The model under review builds one solid part; all positions refer to its coordinate system, in mm. A direction names the side the tool comes from. Round coordinates to 2 decimals unless told otherwise and drop trailing zeros. Order: outer loops, then holes, each group sorted by start corner. A loop starts at its lowest first (then second) coordinate and runs counter-clockwise, first axis right, second up.
1) Machinability: for faces 5 (the face through (1, -9.565, 15)), 6 (the face through (1, -2.785, 3)), 7 (the face through (-31, 7, 9.2)), which of the approach directions +Z, -Z, +X, -X, +Y, -Y give a long, thin tool a straight path to every point of the face, cutting with its end or side? Answer none if there is none.
2) Mouldability with a two-part tool opening along Z and no side actions: class faces 1 (the face through (-29.861, 7, 9)), 2 (the face through (-0.03, -10.07, -0.49)), 3 (the face through (1, 23.495, 10)), 4 (the face through (22.512, 15.613, 9.986)) as pulls with the +Z half, pulls with the -Z half, needs draft (parallel to the pull), parting line crosses it, or undercut.
3) To check wall thickness, follow L1, parallel to X at y = -1.5, z = 8.25; L2, parallel to Y at x = 1, z = 9.75; L3, parallel to Y at x = 16.5, z = 15.75. State the ranges of each line that lie inside material, in increasing order.
4) Consider section B-B (z = 8.2). Give the boundary of the cut face in (x, y).
5) Clearance check with flat-ended pins moving along their axes: P1, Ø1.2, axis at x = -31, y = 10, coming from the +Z side; P2, Ø1, axis at y = 3, z = 15, coming from the +X side; P3, Ø4.5, axis at x = -23, y = 16.5, coming from the +Z side. State where each tip first meets the part, or that it passes through.
6) Consider section D-D (z = 3.75). Give the boundary of the cut face in (x, y) (3 decimals).
Autodesk Inventor part; units mm, degrees
ref_plane "YZ Plane" through (0, 0, 0) normal (1, 0, 0) x (0, 1, 0)
ref_plane "XZ Plane" through (0, 0, 0) normal (0, 1, 0) x (-1, 0, 0)
ref_plane "XY Plane" through (0, 0, 0) normal (0, 0, 1) x (1, 0, 0)
sketch "Sketch1" plane through (0, 0, 0) normal (0, 0, 1) x (1, 0, 0)
  line L0 (-31.3608, 24.9952) -> (32.1392, 24.9952)
  line L1 (32.1392, 24.9952) -> (32.1392, -10.5648)
  line L2 (32.1392, -10.5648) -> (-31.3608, -10.5648)
  line L3 (-31.3608, -10.5648) -> (-31.3608, 24.9952)
  line L4 (30.6392, 23.4952) -> (-29.8608, 23.4952)
  line L5 (-29.8608, 23.4952) -> (-29.8608, -9.0648)
  line L6 (-29.8608, -9.0648) -> (30.6392, -9.0648)
  line L7 (30.6392, -9.0648) -> (30.6392, 23.4952)
  point P0 (0, 0)
  dimension "d0" = 63.5
  dimension "d1" = 35.56
  dimension "d2" = 1.5
extrude "Extrusion1" add sketch "Sketch1" along normal blind 16.2
sketch "Sketch2" plane through (0, 0, 0) normal (0, 0, -1) x (-1, 0, 0)
  line L0 (-32.1392, -10.5648) -> (31.3608, -10.5648)
  line L1 (31.3608, -10.5648) -> (31.3608, 24.9952)
  line L2 (31.3608, 24.9952) -> (-32.1392, 24.9952)
  line L3 (-32.1392, 24.9952) -> (-32.1392, -10.5648)
  point P0 (0, 0)
extrude "Extrusion2" add sketch "Sketch2" along normal blind 1.5
sketch "Sketch3" plane through (0, 0, 0) normal (0, 0, 1) x (1, 0, 0)
  line L0 (-18.6108, 17.2152) -> (19.3892, 17.2152)
  line L1 (19.3892, 17.2152) -> (19.3892, -2.7848)
  line L2 (19.3892, -2.7848) -> (-18.6108, -2.7848)
  line L3 (-18.6108, -2.7848) -> (-18.6108, 17.2152)
  line L4 (30.6392, -9.0648) -> (-29.8608, -9.0648)
  line L5 (-29.8608, 23.4952) -> (30.6392, 23.4952)
  line L6 (30.6392, 23.4952) -> (30.6392, -9.0648)
  line L7 (30.6392, -9.0648) -> (30.6392, 23.4952)
  line L8 (30.6392, 23.4952) -> (-29.8608, 23.4952)
  line L9 (-29.8608, 23.4952) -> (-29.8608, -9.0648)
  line L10 (-29.8608, -9.0648) -> (30.6392, -9.0648)
  point P0 (0, 0)
  dimension "d7" = 38
  dimension "d8" = 20
  dimension "d9" = 6.28
  dimension "d10" = 32.56
  dimension "d11" = 11.25
  dimension "d12" = 60.5
extrude "Extrusion3" add sketch "Sketch3" along normal blind 6
sketch "Sketch4" plane through (0, 0, 6) normal (0, 0, 1) x (1, 0, 0)
  circle A0 centre (-22.4708, 16.1052) radius 1
  circle A1 centre (-22.4708, -1.6748) radius 1
  circle A2 centre (23.2492, -1.6748) radius 1
  circle A3 centre (23.2489, 16.2887) radius 1
  line L0 (30.6392, -9.0648) -> (-29.8608, -9.0648)
  line L1 (-29.8608, 23.4952) -> (30.6392, 23.4952)
  line L2 (-29.8608, -9.0648) -> (-29.8608, 23.4952)
  point P0 (0, 0)
  dimension "d15" = 2
  dimension "d16" = 2
  dimension "d17" = 2
  dimension "d18" = 2
  dimension "d19" = 45.72
  dimension "d20" = 45.72
  dimension "d21" = 17.78
  dimension "d22" = 7.39
  dimension "d23" = 32.56
  dimension "d24" = 60.5
  dimension "d25" = 7.39
  dimension "d26" = 0
extrude "Extrusion4" add sketch "Sketch4" along normal blind 5
sketch "Sketch5" plane through (0, 0, 6) normal (0, 0, 1) x (1, 0, 0)
  circle A0 centre (-22.4708, 16.1052) radius 1
  circle A1 centre (-22.4708, -1.6748) radius 1
  circle A2 centre (23.2492, -1.6748) radius 1
  circle A3 centre (23.2489, 16.2887) radius 1
  circle A4 centre (-22.4708, 16.1052) radius 2
  circle A5 centre (-22.4708, -1.6748) radius 2
  circle A6 centre (23.2492, -1.6748) radius 2
  circle A7 centre (23.2489, 16.2887) radius 2
  point P0 (0, 0)
  dimension "d29" = 1
  dimension "d30" = 1
  dimension "d31" = 1
  dimension "d32" = 1
extrude "Extrusion5" add sketch "Sketch5" along normal blind 3
fillet "Fillet1" radius 1.5 4 edges at (-31.3608, -10.5648, 7.35) (32.1392, -10.5648, 7.35) (32.1392, 24.9952, 7.35) (-31.3608, 24.9952, 7.35)
sketch "Sketch6" plane through (32.1392, -9.0648, 16.2) normal (1, 0, 0) x (0, 0, -1)
  circle A0 centre (8, 16.28) radius 3.2
  line L0 (0, 0) -> (0, 32.56)
  line L1 (0, -1.5) -> (17.7, -1.5)
  line L2 (17.7, 34.06) -> (0, 34.06)
  point P0 (16.2, 9.0648)
  dimension "d36" = 6.4
  dimension "d37" = 8
  dimension "d38" = 17.78
  dimension "d39" = 35.56
extrude "Extrusion6" cut sketch "Sketch6" against normal up to surface (12.75 mm away)
sketch "Sketch7" plane through (19.3892, -2.7848, 0) normal (-1, 0, 0) x (0, 0, 1)
  arc A0 (6, 12.3238) -> (6, 7.6762) centre (8.2, 10) ccw
  circle A1 centre (8.2, 10) radius 5.5
  point P0 (0, 2.7848)
  dimension "d42" = 11
extrude "Extrusion7" cut sketch "Sketch7" against normal up to surface (11.25 mm away)
sketch "Sketch8" plane through (0, 0, 6) normal (0, 0, 1) x (1, 0, 0)
  line L0 (-18.6108, -2.7848) -> (-18.6108, 17.2152)
  line L1 (-18.6108, 2.4694) -> (-22.595, 2.4694)
  line L2 (-22.595, 2.4694) -> (-22.595, 12.7792)
  line L3 (-22.595, 12.7792) -> (-18.6108, 12.7792)
  line L4 (-18.6108, 12.7792) -> (-18.6108, 2.4694)
  point P0 (0, 0)
extrude "Extrusion8" cut sketch "Sketch8" against normal up to surface (6 mm away)
chamfer "Chamfer1" distance 2 angle 45 2 edges at (-18.6108, 2.4694, 3) (-18.6108, 12.7792, 3)
chamfer "Chamfer2" distance 4 angle 45 1 edges at (-22.595, 7.6243, 6)
sketch "Sketch9" plane through (0, 0, 16.2) normal (0, 0, 1) x (1, 0, 0)
  line L0 (-29.8608, 23.4952) -> (30.6392, 23.4952)
  line L1 (-29.8608, -9.0648) -> (-29.8608, 23.4952)
  line L2 (30.6392, -9.0648) -> (-29.8608, -9.0648)
  line L3 (30.6392, 23.4952) -> (30.6392, -9.0648)
  line L4 (29.6392, 22.4952) -> (-28.8608, 22.4952)
  line L5 (-28.8608, 22.4952) -> (-28.8608, -8.0648)
  line L6 (-28.8608, -8.0648) -> (29.6392, -8.0648)
  line L7 (29.6392, -8.0648) -> (29.6392, 22.4952)
  point P0 (0, 0)
  dimension "d53" = 1
extrude "Extrusion9" add sketch "Sketch9" against normal blind 3
chamfer "Chamfer3" distance 1 angle 45 4 edges at (-28.8608, 7.2152, 13.2) (0.3892, 22.4952, 13.2) (0.3892, -8.0648, 13.2) (29.6392, 7.2152, 13.2)
sketch "Sketch10" plane through (0, 0, 16.2) normal (0, 0, 1) x (1, 0, 0)
  line L0 (30.6392, 24.9952) -> (-29.8608, 24.9952)
  arc A0 (-29.8608, 24.9952) -> (-31.3608, 23.4952) centre (-29.8608, 23.4952) ccw
  line L1 (-31.3608, 23.4952) -> (-31.3608, -9.0648)
  arc A1 (-31.3608, -9.0648) -> (-29.8608, -10.5648) centre (-29.8608, -9.0648) ccw
  line L2 (-29.8608, -10.5648) -> (30.6392, -10.5648)
  arc A2 (30.6392, -10.5648) -> (32.1392, -9.0648) centre (30.6392, -9.0648) ccw
  line L3 (32.1392, -9.0648) -> (32.1392, 23.4952)
  arc A3 (32.1392, 23.4952) -> (30.6392, 24.9952) centre (30.6392, 23.4952) ccw
  line L4 (-29.8608, 23.9952) -> (30.6392, 23.9952)
  arc A4 (31.1392, 23.4952) -> (30.6392, 23.9952) centre (30.6392, 23.4952) ccw
  line L5 (31.1392, 23.4952) -> (31.1392, -9.0648)
  arc A5 (30.6392, -9.5648) -> (31.1392, -9.0648) centre (30.6392, -9.0648) ccw
  line L6 (30.6392, -9.5648) -> (-29.8608, -9.5648)
  arc A6 (-30.3608, -9.0648) -> (-29.8608, -9.5648) centre (-29.8608, -9.0648) ccw
  line L7 (-30.3608, -9.0648) -> (-30.3608, 23.4952)
  arc A7 (-29.8608, 23.9952) -> (-30.3608, 23.4952) centre (-29.8608, 23.4952) ccw
  point P0 (0, 0)
  dimension "d59" = 1
extrude "Extrusion10" cut sketch "Sketch10" against normal blind 2
sketch "Sketch11" plane through (-31.3608, -9.0648, -1.5) normal (-1, 0, 0) x (0, 0, 1)
  line L0 (17.7, 32.56) -> (17.7, 0)
  line L1 (10.7, 22.06) -> (17.7, 22.06)
  line L2 (17.7, 22.06) -> (17.7, 10.5)
  line L3 (17.7, 10.5) -> (10.7, 10.5)
  line L4 (10.7, 10.5) -> (10.7, 22.06)
  line L5 (15.7, 34.06) -> (0, 34.06)
  line L6 (0, -1.5) -> (15.7, -1.5)
  point P0 (1.5, 9.0648)
  dimension "d62" = 12
  dimension "d63" = 12
  dimension "d64" = 7
extrude "Extrusion11" cut sketch "Sketch11" against normal up to surface (2.5 mm away)
chamfer "Chamfer4" distance 1 distance2 2 8 edges at (0.3892, -10.5648, -1.5) (-30.9214, -10.1255, -1.5) (-31.3608, 7.2152, -1.5) (-30.9214, 24.5559, -1.5) (0.3892, 24.9952, -1.5) (31.6999, 24.5559, -1.5) (32.1392, 7.2152, -1.5) (31.6999, -10.1255, -1.5) measured on face at (-9.6941, 13.1419, -1.5)
equation "\"d9\" = -0.5 * d8 + 0.5 * d10"
equation "\"d11\" = -0.5 * d7 + 0.5 * d12"
equation "\"d20\" = d19"
equation "\"d22\" = -0.5 * d21 + 0.5 * d23"
equation "\"d25\" = -0.5 * d19 + 0.5 * d24"
equation "\"d38\" = 0.5 * d39"
properties part number "NodeEnclosure"
Answer below:
1. face 5: +Z, +X, -X, -Y
1. face 6: +Z
1. face 7: +Z, -X
2. face 1: undercut
2. face 2: pulls with the -Z half
2. face 3: undercut
2. face 4: needs draft
3. L1: x = -31.36 to -29.86, -24.46 to -20.48, 21.26 to 25.24, 30.64 to 32.14
3. L2: y = -10.56 to -9.06, 23.5 to 25
3. L3: y = -9.56 to -8.06, 22.5 to 24
4. outline: (-31.36, -9.06) arc R1.5 ccw to (-29.86, -10.56) - (30.64, -10.56) arc R1.5 ccw to (32.14, -9.06) - (32.14, 4.02) - (30.64, 4.02) - (30.64, -9.06) - (-29.86, -9.06) - (-29.86, 23.5) - (30.64, 23.5) - (30.64, 10.42) - (32.14, 10.42) - (32.14, 23.5) arc R1.5 ccw to (30.64, 25) - (-29.86, 25) arc R1.5 ccw to (-31.36, 23.5) - close; circle Ø4 at (-22.47, -1.67); circle Ø4 at (-22.47, 16.11); circle Ø4 at (23.25, -1.67); circle Ø4 at (23.25, 16.29)
5. P1: stops at z = 9.2
5. P2: stops at x = 31.14
5. P3: stops at z = 11
6. outline: (-31.361, -9.065) arc R1.5 ccw to (-29.861, -10.565) - (30.639, -10.565) arc R1.5 ccw to (32.139, -9.065) - (32.139, 23.495) arc R1.5 ccw to (30.639, 24.995) - (-29.861, 24.995) arc R1.5 ccw to (-31.361, 23.495) - close; hole (-24.345, 2.469) - (-20.611, 2.469) - (-18.611, 0.469) - (-18.611, -2.785) - (19.389, -2.785) - (19.389, 3.983) - (30.639, 3.983) - (30.639, 10.447) - (19.389, 10.447) - (19.389, 17.215) - (-18.611, 17.215) - (-18.611, 14.779) - (-20.611, 12.779) - (-24.345, 12.779) - close
